```python
from build123d import *
from build123d.topology import SkipClean

# Parameters (mm, degrees)
SKETCH1_R           = 22
BOSS_EXTRUDE1_DEPTH = 17.6
SKETCH2_R           = 15
CUT_EXTRUDE1_DEPTH  = 3.6
CUT_EXTRUDE2_DEPTH  = 37.18
BOSS_EXTRUDE2_START = 0.45
SKETCH4_R           = 15
SKETCH4_R_2         = 11
SKETCH4_R_3         = 3.35
BOSS_EXTRUDE2_DEPTH = 0.45
SKETCH5_R           = 10.75
CUT_EXTRUDE3_DEPTH  = 9
FILLET1_R           = 4


with BuildPart() as part:
    # Sketch1 → Boss-Extrude1 (new body)
    with BuildSketch(Plane(origin=(0, 0, 0), x_dir=(1, 0, 0), z_dir=(0, 1, 0))):
        with Locations(Location((0, 0, 0), (0, 0, 270))):
            Circle(SKETCH1_R)
    extrude(amount=BOSS_EXTRUDE1_DEPTH)

    # Sketch2 → Cut-Extrude1 (cut)
    with BuildSketch(Plane(origin=(0, 17.6, 0), x_dir=(1, 0, 0), z_dir=(0, 1, 0))):
        with Locations(Location((0, 0, 0), (0, 0, 270))):
            Circle(SKETCH2_R)
    extrude(amount=-CUT_EXTRUDE1_DEPTH, mode=Mode.SUBTRACT)

    # Sketch3 → Cut-Extrude2 (cut)
    with BuildSketch(Plane(origin=(0, 14, 0), x_dir=(1, 0, 0), z_dir=(0, 1, 0))):
        with BuildLine():
            ThreePointArc((1.4, 0), (-0.448663748, 1.326160187), (-1.112429773, -0.85))
            Line((-1.112429773, -0.85), (1.112429773, -0.85))
            ThreePointArc((1.112429773, -0.85), (1.326160187, -0.448663748), (1.4, 0))
        make_face()
    extrude(amount=-CUT_EXTRUDE2_DEPTH, mode=Mode.SUBTRACT)

    # Sketch4 → Boss-Extrude2 (add)
    # profile 1 of 2: a face of its own
    with SkipClean():  # the faces are left unmerged after this step: merging them gives an invalid solid
        with BuildSketch(Plane(origin=(0, 14, 0), x_dir=(1, 0, 0), z_dir=(0, 1, 0)).offset(BOSS_EXTRUDE2_START)):
            with Locations(Location((0, 0, 0), (0, 0, 270))):
                Circle(SKETCH4_R)
            with Locations(Location((0, 0, 0), (0, 0, 270))):
                Circle(SKETCH4_R_2, mode=Mode.SUBTRACT)
        # profile 2 of 2: a face of its own
        with BuildSketch(Plane(origin=(0, 14, 0), x_dir=(1, 0, 0), z_dir=(0, 1, 0)).offset(BOSS_EXTRUDE2_START)):
            with Locations(Location((0, 0, 0), (0, 0, 270))):
                Circle(SKETCH4_R_3)
            with BuildLine():
                Line((1.112429773, -0.85), (-1.112429773, -0.85))
                ThreePointArc((-1.112429773, -0.85), (0, 1.4), (1.112429773, -0.85))
            make_face(mode=Mode.SUBTRACT)
        extrude(amount=-BOSS_EXTRUDE2_DEPTH)

    # Sketch5 → Cut-Extrude3 (cut)
    with SkipClean():  # the faces are left unmerged after this step: merging them gives an invalid solid
        with BuildSketch(Plane.XZ):
            with Locations(Location((0, 0, 0), (0, 0, 270))):
                Circle(SKETCH5_R)
        extrude(amount=-CUT_EXTRUDE3_DEPTH, mode=Mode.SUBTRACT)

    # Fillet1
    fillet1_edges = [part.edges().sort_by_distance(p)[0] for p in [
        (0, 0, -22),
        (0, 17.6, -22),
    ]]
    fillet(fillet1_edges, radius=FILLET1_R)


solid = part.part
```
Here's how the part is built. I have some questions about the finished solid (model axes, mm). A direction names the side the tool comes from. Coordinates: 2 decimals unless noted, no trailing zeros. Order: outer loops, then holes, each group sorted by start corner. A loop starts at its lowest first (then second) coordinate and runs counter-clockwise, first axis right, second up. Notation, with made-up numbers: (56.5, 88) - (110.5, 88) arc R22 ccw to (110.5, 118) - close; hole circle Ø10 at (77.25, -19.75). An arc over 180 degrees is marked (long way). One line per question, with ' | ' between items.
(1) Suppose I cut it at A-A on x = 0. List the corners of the cut face in (y, z) for me.
Report:
outline: (0, -18) arc R4 ccw to (4, -22) - (13.6, -22) arc R4 ccw to (17.6, -18) - (17.6, -15) - (14.45, -15) - (14.45, -11) - (14, -11) - (14, -3.35) - (14.45, -3.35) - (14.45, -1.4) - (9, -1.4) - (9, -10.75) - (0, -10.75) - close; (0, 10.75) - (9, 10.75) - (9, 0.85) - (14.45, 0.85) - (14.45, 3.35) - (14, 3.35) - (14, 11) - (14.45, 11) - (14.45, 15) - (17.6, 15) - (17.6, 18) arc R4 ccw to (13.6, 22) - (4, 22) arc R4 ccw to (0, 18) - close
(2) For faces 4 (the flat face through (15, 17.6, -4)), 5 (the cylindrical face through (7.27, 4.44, 7.92)), 6 (the flat face through (0, 12, 0.85)), 7 (the cylindrical face through (0.66, 16.047, -14.985)), which set-ups out of +Z, -Z, +X, -X, +Y, -Y let a thin tool reach every point of the face, with its end or its side?
Report:
face 4: +Z, -Z, +X, -X, +Y | face 5: -Y | face 6: +Y, -Y | face 7: +Y
(3) If I drill on L1, parallel to X at y = 14.25, z = 0; L2, parallel to Y at x = -3, z = -12; L3, parallel to X at y = 15, z = 2, over which ranges is the centre line in solid material (lowest first)?
Report:
L1: x = -21.95 to -11, -3.35 to -1.4, 1.4 to 3.35, 11 to 21.95 | L2: y = 0 to 14.45 | L3: x = -21.65 to -14.87, 14.87 to 21.65
(4) If we mould it in two halves opening along X, with no side actions, what happens to faces 1 (the flat face through (-8, 0, 8)), 2 (the cylindrical face through (-21.477, 8.733, -4.769)), 3 (the flat face through (10, 14.45, -5))? For each: pulls with the +X half, pulls with the -X half, needs draft (parallel to the pull), parting line crosses it, or undercut.
Report:
face 1: needs draft | face 2: parting line crosses it | face 3: undercut
(5) Suppose I cut it at D-D on y = 2. List the corners of the cut face in (x, z) for me, and give its area (3 significant figures).
Report:
outline: circle Ø42.93 at (0, 0); hole circle Ø21.5 at (0, 0) | area: 1,080 mm2
(6) Suppose I cut it at B-B on y = 7. List the corners of the cut face in (x, z) for me.
Report:
outline: circle Ø44 at (0, 0); hole circle Ø21.5 at (0, 0)
(7) Will these pins go through, and if not, where does the flat tip stop? pin 1 (6 mm diameter, centred on x = -8, y = 13, fed in from +Z); pin 2 (9 mm diameter, centred on x = -6.5, z = 5, fed in from +Y); pin 3 (12 mm diameter, centred on x = -4.5, z = 3.5, fed in from -Y); pin 4 (1 mm diameter, centred on y = 8, z = -12, fed in from -X) (3 decimals).
Report:
pin 1: stops at z = 21.42 | pin 2: stops at y = 14.45 | pin 3: stops at y = 0 | pin 4: stops at x = -18.755
(8) Suppose I cut it at C-C on y = 10. List the corners of the cut face in (x, z) for me, and give its area (3 significant figures).
Report:
outline: circle Ø44 at (0, 0); hole (-1.11, 0.85) arc R1.4 ccw (long way) to (1.11, 0.85) - close | area: 1,520 mm2
